```python
from build123d import *

# Parameters (mm, degrees)
BOSS_EXTRUDE1_DEPTH      = 65
BOSS_EXTRUDE1_DEPTH_BACK = 65
BOSS_EXTRUDE2_DEPTH      = 12
FILLET1_R                = 10
FILLET2_R                = 10


with BuildPart() as part:
    # Sketch1 → Boss-Extrude1 (new, two sides: drawn at the far end of the back side and taken through both)
    with BuildSketch(Plane.XY.offset(-BOSS_EXTRUDE1_DEPTH_BACK)):
        with BuildLine():
            Line((-11.3, 11.7), (11.3, 11.7))
            ThreePointArc((11.3, 11.7), (23, 0), (11.3, -11.7))
            Line((11.3, -11.7), (-11.3, -11.7))
            ThreePointArc((-11.3, -11.7), (-23, 0), (-11.3, 11.7))
        make_face()
    extrude(amount=BOSS_EXTRUDE1_DEPTH + BOSS_EXTRUDE1_DEPTH_BACK)

    # Sketch2 → Boss-Extrude2 (add)
    with BuildSketch(Plane.XY.offset(65)):
        with BuildLine():
            Line((-11.3, 12.2), (11.3, 12.2))
            ThreePointArc((11.3, 12.2), (23.5, 0), (11.3, -12.2))
            Line((11.3, -12.2), (-11.3, -12.2))
            ThreePointArc((-11.3, -12.2), (-23.5, 0), (-11.3, 12.2))
        make_face()
    boss_extrude2 = extrude(amount=-BOSS_EXTRUDE2_DEPTH)

    # Mirror1: Boss-Extrude2 across plane
    add(boss_extrude2.mirror(Plane.XY))

    # Fillet1
    # the kernel refuses this fillet: 10 mm, written as the material it adds along each edge
    with BuildSketch(Plane(origin=(-11.3, -11.7, 53), x_dir=(0, -1.0, -2.188471626126437e-12), z_dir=(1, 0, 0)), Plane(origin=(11.3, 11.7, 53), x_dir=(0, 1.0, -2.188471626126375e-12), z_dir=(-1, 0, 0))) as fillet1_piece_1:
        with BuildLine():
            CenterArc((10, 3.122498999), FILLET1_R, 180, 18.194872339)
            Line((0, 3.122498999), (-0.2, 3.122498999))
            Line((-0.2, 3.122498999), (-0.2, 0))
            Line((-0.2, 0), (0, -0.2))
            ThreePointArc((0, -0.2), (0.25, -0.2), (0.31, -0.06244998))
            Line((0.31, -0.06244998), (0.5, 0))
        make_face()
    extrude(amount=22.6)
    with BuildSketch(Plane(origin=(-11.3, 0, 53), x_dir=(0, -1, 0), z_dir=(1, 0, 0))) as fillet1_piece_2:
        with BuildLine():
            CenterArc((21.7, 3.122498999), FILLET1_R, 180, 18.194872339)
            Line((11.7, 3.122498999), (11.5, 3.122498999))
            Line((11.5, 3.122498999), (11.5, 0))
            Line((11.5, 0), (11.7, -0.2))
            ThreePointArc((11.7, -0.2), (11.95, -0.2), (12.01, -0.06244998))
            Line((12.01, -0.06244998), (12.2, 0))
        make_face()
    revolve(axis=Axis((-11.3, 0, 53), (0, 0, -1)), revolution_arc=180)
    with BuildSketch(Plane(origin=(11.3, 0, 53), x_dir=(0, 1, 0), z_dir=(-1, 0, 0))) as fillet1_piece_3:
        with BuildLine():
            CenterArc((21.7, 3.122498999), FILLET1_R, 180, 18.194872339)
            Line((11.7, 3.122498999), (11.5, 3.122498999))
            Line((11.5, 3.122498999), (11.5, 0))
            Line((11.5, 0), (11.7, -0.2))
            ThreePointArc((11.7, -0.2), (11.95, -0.2), (12.01, -0.06244998))
            Line((12.01, -0.06244998), (12.2, 0))
        make_face()
    revolve(axis=Axis((11.3, 0, 53), (0, 0, -1)), revolution_arc=180)

    # Fillet2
    # the kernel refuses this fillet: 10 mm, written as the material it adds along each edge
    with BuildSketch(Plane(origin=(-11.3, -11.7, -53), x_dir=(0, -1.0, 2.188471626126437e-12), z_dir=(1, 0, 0))) as fillet2_piece_1:
        with BuildLine():
            CenterArc((10, -3.122498999), FILLET2_R, 161.805127661, 18.194872339)
            Line((0, -3.122498999), (-0.2, -3.122498999))
            Line((-0.2, -3.122498999), (-0.2, 0))
            Line((-0.2, 0), (0, 0.2))
            ThreePointArc((0, 0.2), (0.25, 0.2), (0.31, 0.06244998))
            Line((0.31, 0.06244998), (0.5, 0))
        make_face()
    extrude(amount=22.6)
    with BuildSketch(Plane(origin=(11.3, 11.7, -53), x_dir=(0, 0, 1), z_dir=(-1, 0, 0))) as fillet2_piece_2:
        with BuildLine():
            CenterArc((3.122498999, 10), FILLET2_R, 251.805127661, 18.194872339)
            Line((0, 0.5), (-0.06244998, 0.31))
            ThreePointArc((-0.06244998, 0.31), (-0.2, 0.25), (-0.2, 0))
            Line((-0.2, 0), (0, -0.2))
            Line((0, -0.2), (3.122498999, -0.2))
            Line((3.122498999, -0.2), (3.122498999, 0))
        make_face()
    extrude(amount=22.6)
    with BuildSketch(Plane(origin=(-11.3, 0, -53), x_dir=(0, -1, 0), z_dir=(1, 0, 0))) as fillet2_piece_3:
        with BuildLine():
            CenterArc((21.7, -3.122498999), FILLET2_R, 161.805127661, 18.194872339)
            Line((11.7, -3.122498999), (11.5, -3.122498999))
            Line((11.5, -3.122498999), (11.5, 0))
            Line((11.5, 0), (11.7, 0.2))
            ThreePointArc((11.7, 0.2), (11.95, 0.2), (12.01, 0.06244998))
            Line((12.01, 0.06244998), (12.2, 0))
        make_face()
    revolve(axis=Axis((-11.3, 0, -53), (0, 0, -1)), revolution_arc=180)
    with BuildSketch(Plane(origin=(11.3, 0, -53), x_dir=(0, 1, 0), z_dir=(-1, 0, 0))) as fillet2_piece_4:
        with BuildLine():
            CenterArc((21.7, -3.122498999), FILLET2_R, 161.805127661, 18.194872339)
            Line((12.2, 0), (12.01, 0.06244998))
            ThreePointArc((12.01, 0.06244998), (11.95, 0.2), (11.7, 0.2))
            Line((11.7, 0.2), (11.5, 0))
            Line((11.5, 0), (11.5, -3.122498999))
            Line((11.5, -3.122498999), (11.7, -3.122498999))
        make_face()
    revolve(axis=Axis((11.3, 0, -53), (0, 0, -1)), revolution_arc=180)


solid = part.part
```
CAD build for the part. Positions are in the model's coordinates, mm. A direction names the side the tool comes from. Round coordinates to 2 decimals unless told otherwise and drop trailing zeros. Loops run counter-clockwise (first coordinate to the right, second up) from the corner with the lowest first, then second, coordinate; pieces in that order, holes last. Notation, with made-up numbers: M 65.5,-13 L 82.5,-13 A26 ccw 82.5,8 Z; hole C 75,55.25 d1. An arc over 180 degrees is marked long. Use a Markdown table: item, result. Add a question column.
(1) Pull direction Z, two halves, no side cores. Call faces 6 (the face through (-23, 0, -1)), 7 (the face through (0, 0, 65)), 8 (the face through (0, 0, -65)), 9 (the face through (-23.497, -0.268, -59.084)): +Z half, -Z half, draft (parallel to the pull), parting line (faces both ways), or undercut.
(2) Drill centre lines: line 1 (Y direction, x = 5, z = 6); line 2 (X direction, y = 7.75, z = -52); line 3 (X direction, y = 4.5, z = 16). Where is each one in solid material? Low to high.
(3) Which spindle directions (+Z, -Z, +X, -X, +Y, -Y) get a long thin tool onto all of the face, cutting with end or side? Do faces 1 (the face through (0, 11.7, -1)), 2 (the face through (0, 12.2, 59)), 3 (the face through (0, -12.2, -59)), 4 (the face through (-0.16, -11.83, -51.48)), 5 (the face through (23, 0, -1)). Say none if no direction does.
(4) Cut at C-C (z = -23). Give the cut face in (x, y).
(5) Cut at B-B (z = 55.5). Give the cut face in (x, y).
(6) Cut at A-A (y = 0). Give the cut face in (x, z), and give its area (3 significant figures).
(7) Flat gauge pins, fed straight in: pin 1 (2 mm diameter, centred on x = -1, z = -18, fed in from +Y); pin 2 (25 mm diameter, centred on x = 3, z = -8.5, fed in from -Y); pin 3 (1.5 mm diameter, centred on x = -16, z = -19.5, fed in from +Y). Where does each tip first touch, or does it go through?
Geometry says:
| question | item | result |
|---|---|---|
| 1 | face 6 | undercut |
| 1 | face 7 | +Z half |
| 1 | face 8 | -Z half |
| 1 | face 9 | draft |
| 2 | line 1 | y = -11.7 to 11.7 |
| 2 | line 2 | x = -20.37 to 20.37 |
| 2 | line 3 | x = -22.1 to 22.1 |
| 3 | face 1 | +X, -X, +Y |
| 3 | face 2 | +Z, -Z, +X, -X, +Y |
| 3 | face 3 | +Z, -Z, +X, -X, -Y |
| 3 | face 4 | +X, -X, -Y |
| 3 | face 5 | +X |
| 4 | outline | M -11.3,-11.7 L 11.3,-11.7 A11.7 ccw 11.3,11.7 L -11.3,11.7 A11.7 ccw Z |
| 5 | outline | M -11.3,-12.2 L 11.3,-12.2 A12.2 ccw 11.3,12.2 L -11.3,12.2 A12.2 ccw Z |
| 6 | outline | M -23.5,-65 L 23.5,-65 L 23.5,-53 A10 cw 23,-49.88 L 23,49.88 A10 cw 23.5,53 L 23.5,65 L -23.5,65 L -23.5,53 A10 cw -23,49.88 L -23,-49.88 A10 cw -23.5,-53 Z |
| 6 | area | 6,010 mm² |
| 7 | pin 1 | stops at y = 11.7 |
| 7 | pin 2 | stops at y = -11.7 |
| 7 | pin 3 | stops at y = 11.01 |
